Could you check a few things on this model? Use its own coordinates, in mm. A direction names the side the tool comes from. Round coordinates to 2 decimals unless told otherwise and drop trailing zeros. Write each loop counter-clockwise with the first axis right and the second up, starting at its lowest first coordinate (ties: lowest second). Pieces come first, ordered by that corner, then holes.
```python
from build123d import *

# Parameters (mm, degrees)
F0_R     = 1.75
F1_DEPTH = 2.5
F2_R     = 2
F3_R     = 2


with BuildPart() as f1:
    # F0 (on Top) → F1 (new body)
    with BuildSketch(Plane.XY):
        Polygon((10, 5), (-5, 5), (-5, -5), (10, -5), (10, -2.5), (3.8, -2.5), (3.8, 2.5), (10, 2.5), align=None)
        Circle(F0_R, mode=Mode.SUBTRACT)
    extrude(amount=F1_DEPTH)

    # F2
    f2_edges = [f1.edges().sort_by_distance(p)[0] for p in [
        (3.8, 2.5, 1.25),
    ]]
    fillet(f2_edges, radius=F2_R)

    # F3
    f3_edges = [f1.edges().sort_by_distance(p)[0] for p in [
        (3.8, -2.5, 1.25),
    ]]
    fillet(f3_edges, radius=F3_R)


solid = f1.part
```
Q1. If I drill on L1, parallel to Y at x = 8.5, z = 1.9; L2, parallel to Y at x = 0, z = 1.7; L3, parallel to X at y = 0.25, z = 0.8, over which ranges is the centre line in solid material (lowest first)?
Q2. Imagine slicing it at B-B, the plane y = 0. Write out the boundary of the cut face in (x, z), then the cut area to 4 significant figures.
Q3. I'm going to push a flat-ended pin straight in: pin 1 Ø3 at (x, y) = (0, 0) entering from +Z. Where does the tip first touch, or does it pass through?
Q4. Imagine slicing it at C-C, the plane z = 0.2. Write out the boundary of the cut face in (x, y).
Q5. We'd pull the mould along X, two halves only. Please class faces 3 (the cylindrical face through (1.617, -0.67, 1.232)), 4 (the flat face through (10, -4, 1)), 5 (the flat face through (3, 5, 1)): pulls with the +X half, pulls with the -X half, needs draft (parallel to the pull), parting line crosses it, or undercut.
Q6. Imagine slicing it at A-A, the plane x = 0. Write out the boundary of the cut face in (y, z).
Q7. On a 3-axis mill with a long thin cutter (end or side, diameter ignored), from which of +Z, -Z, +X, -X, +Y, -Y can I reach the whole of each face in a straight line? I mean faces 1 (the cylindrical face through (4.37, -1.9, 1.27)), 2 (the flat face through (2, -5, 1)). Say none if no direction works.
Results found:
1. L1: y = -5 to -2.5, 2.5 to 5
1. L2: y = -5 to -1.75, 1.75 to 5
1. L3: x = -5 to -1.73, 1.73 to 3.8
2. outline: (-5, 0) - (-1.75, 0) - (-1.75, 2.5) - (-5, 2.5) - close; (1.75, 0) - (3.8, 0) - (3.8, 2.5) - (1.75, 2.5) - close
2. area: 13.25 mm2
3. pin 1: passes through
4. outline: (-5, -5) - (10, -5) - (10, -2.5) - (5.8, -2.5) arc R2 cw to (3.8, -0.5) - (3.8, 0.5) arc R2 cw to (5.8, 2.5) - (10, 2.5) - (10, 5) - (-5, 5) - close; hole circle Ø3.5 at (0, 0)
5. face 3: undercut
5. face 4: pulls with the +X half
5. face 5: needs draft
6. outline: (-5, 0) - (-1.75, 0) - (-1.75, 2.5) - (-5, 2.5) - close; (1.75, 0) - (5, 0) - (5, 2.5) - (1.75, 2.5) - close
7. face 1: +Z, -Z, +X
7. face 2: +Z, -Z, +X, -X, -Y
